from build123d import *

# Parameters (mm, degrees)
SKETCH1_R           = 5
BOSS_EXTRUDE1_DEPTH = 12
SKETCH2_R           = 5
BOSS_EXTRUDE2_DEPTH = 12
BOSS_EXTRUDE3_DEPTH = 48
FILLET1_R           = 30
SKETCH6_R           = 10
CUT_EXTRUDE1_DEPTH  = 61
SKETCH7_W           = 16
SKETCH7_H           = 3
CUT_EXTRUDE2_DEPTH  = 61
CUT_EXTRUDE3_REACH  = 102
SKETCH9_R           = 6
RIB9_REACH          = 62
SKETCH8_WALL_W      = 167.694197534
SKETCH8_WALL_H      = 8


with BuildPart() as part:
    # Sketch1 → Boss-Extrude1 (new body)
    with BuildSketch(Plane.XY):
        with BuildLine():
            Line((10, 100), (110, 100))
            Line((110, 100), (110, 85))
            Line((110, 85), (95, 85))
            Line((95, 85), (95, 73))
            ThreePointArc((95, 73), (70.911840902, 50.882552147), (62, 19.418286702))
            Line((62, 19.418286702), (62, 0))
            Line((62, 0), (0, 0))
            Line((0, 0), (0, 90))
            ThreePointArc((0, 90), (2.928932188, 97.071067812), (10, 100))
        make_face()
        with Locations((10, 90)):
            Circle(SKETCH1_R, mode=Mode.SUBTRACT)
    extrude(amount=BOSS_EXTRUDE1_DEPTH)

    # Sketch2 → Boss-Extrude2 (add)
    with BuildSketch(Plane.XZ):
        with BuildLine():
            Line((62, 12), (62, 48))
            Line((62, 48), (12, 48))
            ThreePointArc((12, 48), (3.514718626, 44.485281374), (0, 36))
            Line((0, 36), (0, 12))
            Line((0, 12), (62, 12))
        make_face()
        with Locations(Location((12, 36, 0), (0, 0, 270))):  # turned: the seam where the file's is
            Circle(SKETCH2_R, mode=Mode.SUBTRACT)
    extrude(amount=-BOSS_EXTRUDE2_DEPTH)

    # Sketch5 → Boss-Extrude3 (add)
    with BuildSketch(Plane.XY.offset(12)):
        with BuildLine():
            Line((32.650648427, 100), (110, 100))
            Line((110, 100), (110, 85))
            Line((110, 85), (74.819347292, 85))
            ThreePointArc((74.819347292, 85), (41.621443501, 58.445811604), (32.650648427, 100))
        make_face()
    extrude(amount=BOSS_EXTRUDE3_DEPTH)

    # Fillet1
    fillet1_edges = [part.edges().sort_by_distance(p)[0] for p in [
        (110, 92.5, 60),
    ]]
    fillet(fillet1_edges, radius=FILLET1_R)

    # Sketch6 → Cut-Extrude1 (cut, through all)
    with BuildSketch(Plane.XY.offset(60)):
        with Locations((50, 82)):
            Circle(SKETCH6_R)
    extrude(amount=-CUT_EXTRUDE1_DEPTH, mode=Mode.SUBTRACT)

    # Sketch7 → Cut-Extrude2 (cut, through all)
    with BuildSketch(Plane.XY.offset(60)):
        with Locations((50, 98.5)):
            Rectangle(SKETCH7_W, SKETCH7_H)
    extrude(amount=-CUT_EXTRUDE2_DEPTH, mode=Mode.SUBTRACT)

    # Sketch9 → Cut-Extrude3 (cut, up to next)
    with BuildSketch(Plane(origin=(0, 100, 0), x_dir=(1, 0, 0), z_dir=(0, 1, 0)), mode=Mode.PRIVATE) as cut_extrude3_sk1:
        with Locations(Location((90, -30, 0), (0, 0, 270))):  # turned: the seam where the file's is
            Circle(SKETCH9_R)
    cut_extrude3_tool1 = extrude(cut_extrude3_sk1.sketch, amount=-CUT_EXTRUDE3_REACH, mode=Mode.PRIVATE) & part.part
    add(cut_extrude3_tool1.solids().sort_by_distance((90, 100, 30))[0], mode=Mode.SUBTRACT)

    # Sketch8 wall → Rib9 (add, up to next)
    with BuildSketch(Plane(origin=(50, 34.5, 51.967357066), x_dir=(0, 0.984807753, 0.173648178), z_dir=(0, -0.173648178, 0.984807753)), mode=Mode.PRIVATE) as rib9_sk1:
        Rectangle(SKETCH8_WALL_W, SKETCH8_WALL_H)
    rib9_tool1 = extrude(rib9_sk1.sketch, amount=-RIB9_REACH, mode=Mode.PRIVATE) - part.part
    add(rib9_tool1.solids().sort_by_distance((50, 34.5, 51.967357066))[0])


solid = part.part
The model under review builds one solid part; all positions refer to its coordinate system, in mm. A direction names the side the tool comes from. Round coordinates to 2 decimals unless told otherwise and drop trailing zeros. Loops run counter-clockwise (first coordinate to the right, second up) from the corner with the lowest first, then second, coordinate; pieces in that order, holes last. Notation, with made-up numbers: (41, -1) -> (71, -1) arc R35 ccw to (71, 31) -> close; hole circle Ø10 at (71, 32.5). An arc over 180 degrees is marked (long way). Write item = value, one per line. Start each with the question number.
Item 1: For faces 5 (the flat face through (46, 35, 30)), 6 (the flat face through (37, 6, 48)), 7 (the flat face through (42, 98, 30)), list the 3-axis set-ups (+Z, -Z, +X, -X, +Y, -Y) from which the entire face can be reached by the end or side of a thin tool; tool diameter is ignored.
Item 2: Mouldability with a two-part tool opening along Y and no side actions: class faces 1 (the flat face through (31, 0, 24)), 2 (the cylindrical face through (8.92, 85.12, 5.92)), 3 (the flat face through (18, 47, 12)), 4 (the flat face through (50, 97, 30)) as released by +Y, released by -Y, zero draft, split by the parting line, or undercut.
Item 3: To check wall thickness, follow L1, parallel to X at y = 4.5, z = 36; L2, parallel to Y at x = 44.5, z = 18.5; L3, parallel to X at y = 15, z = 19. State the ranges of each line that lie inside material, in increasing order.
Item 4: Insertion check: pin 1 (23 mm diameter, centred on x = 50, y = 82, fed in from +Z); pin 2 (1.5 mm diameter, centred on y = 99, z = 34, fed in from -X); pin 3 (8 mm diameter, centred on x = 12, z = 36, fed in from -Y) (1 decimal); pin 4 (2 mm diameter, centred on y = 20, z = 18, fed in from -X). Each pin has a flat end and moves straight along its axis. Give the tip position at first contact, or say it passes through.
Item 5: Take a section at B-B on x = 50. Give the boundary of the cut face in (y, z).
Item 6: Take a section at D-D on x = 27. Give the boundary of the cut face in (y, z).
Item 7: Take a section at C-C on z = 50.5. Give the boundary of the cut face in (x, y), plus the area to 3 significant figures.
Item 8: Take a section at A-A on y = 82. Give the boundary of the cut face in (x, z).
Result:
q1.face_5 = +Z, -X
q1.face_6 = +Z, +X, -X, -Y
q1.face_7 = +Z, -Z, +Y
q2.face_1 = released by -Y
q2.face_2 = undercut
q2.face_3 = undercut
q2.face_4 = released by +Y
q3.L1 = 0 to 7, 17 to 62
q3.L2 = 0 to 12, 57.61 to 73.65, 90.35 to 97
q3.L3 = 46 to 54
q4.pin_1 = 60
q4.pin_2 = 31
q4.pin_3 = through
q4.pin_4 = 46
q5.outline = (0, 0) -> (72, 0) -> (72, 60) -> (57, 60) -> (57, 55.93) -> (12, 48) -> (0, 48) -> close; (92, 0) -> (97, 0) -> (97, 60) -> (92, 60) -> close
q6.outline = (0, 0) -> (100, 0) -> (100, 12) -> (91.8, 12) -> (91.8, 60) -> (72.2, 60) -> (72.2, 12) -> (12, 12) -> (12, 48) -> (0, 48) -> close
q7.outline = (32.65, 100) arc R25 ccw to (46, 57.32) -> (46, 26.18) -> (54, 26.18) -> (54, 57.32) arc R25 ccw to (74.82, 85) -> (101.9, 85) -> (101.9, 100) -> (58, 100) -> (58, 97) -> (42, 97) -> (42, 100) -> close; hole circle Ø20 at (50, 82)
q7.area = 2,130 mm²
q8.outline = (0, 0) -> (40, 0) -> (40, 60) -> (25, 60) -> (25, 12) -> (0, 12) -> close; (60, 0) -> (95, 0) -> (95, 12) -> (75, 12) -> (75, 60) -> (60, 60) -> close
